from build123d import *

# Parameters (mm, degrees)
SALIENTE_EXTRUIR1_DEPTH = 5
REDONDEO1_R             = 10
CROQUIS2_R              = 1.5
CROQUIS2_W              = 40
CROQUIS2_H              = 20
CORTAR_EXTRUIR1_DEPTH   = 135.669558943
CROQUIS3_W              = 4
CROQUIS3_H              = 14.636342218
CORTAR_EXTRUIR2_DEPTH   = 135.669558943


with BuildPart() as part:
    # Croquis1 → Saliente-Extruir1 (new body)
    with BuildSketch(Plane(origin=(0, 0, 0), x_dir=(1, 0, 0), z_dir=(0, 1, 0))):
        Polygon((-88.1, 42.318171109), (88.1, 42.318171109), (108.1, 22.318171109), (127.75, 22.318171109), (127.75, 7.681828891), (105.75, 7.681828891), (77.75, -42.318171109), (-77.75, -42.318171109), (-105.75, 7.681828891), (-127.75, 7.681828891), (-127.75, 22.318171109), (-108.1, 22.318171109), align=None)
    extrude(amount=SALIENTE_EXTRUIR1_DEPTH)

    # Redondeo1
    redondeo1_edges = [part.edges().sort_by_distance(p)[0] for p in [
        (-88.1, 2.5, -42.318171109),
        (88.1, 2.5, -42.318171109),
        (108.1, 2.5, -22.318171109),
        (105.75, 2.5, -7.681828891),
        (77.75, 2.5, 42.318171109),
        (-77.75, 2.5, 42.318171109),
        (-105.75, 2.5, -7.681828891),
        (-108.1, 2.5, -22.318171109),
    ]]
    fillet(redondeo1_edges, radius=REDONDEO1_R)

    # Croquis2 → Cortar-Extruir1 (cut, through all)
    with BuildSketch(Plane(origin=(0, 5, 0), x_dir=(1, 0, 0), z_dir=(0, 1, 0))):
        with Locations(Location((70, -17.318171109, 0), (0, 0, 270))):
            Circle(CROQUIS2_R)
        with Locations(Location((-70, -17.318171109, 0), (0, 0, 270))):
            Circle(CROQUIS2_R)
        with Locations(Location((-119.996067812, 15, 0), (0, 0, 270))):
            Circle(CROQUIS2_R)
        with Locations(Location((119.996067812, 15, 0), (0, 0, 270))):
            Circle(CROQUIS2_R)
        with Locations(Location((-75, 32.318171109, 0), (0, 0, 270))):
            Circle(CROQUIS2_R)
        with Locations(Location((75, 32.318171109, 0), (0, 0, 270))):
            Circle(CROQUIS2_R)
        with Locations(Location((-10, -22.318171109, 0), (0, 0, 270))):
            Circle(CROQUIS2_R)
        with Locations(Location((10, -22.318171109, 0), (0, 0, 270))):
            Circle(CROQUIS2_R)
        with Locations(Location((-10, -37.318171109, 0), (0, 0, 270))):
            Circle(CROQUIS2_R)
        with Locations(Location((10, -37.318171109, 0), (0, 0, 270))):
            Circle(CROQUIS2_R)
        with Locations(Location((-60, -2.681828891, 0), (0, 0, 270))):
            Circle(CROQUIS2_R)
        with Locations(Location((-10, -2.681828891, 0), (0, 0, 270))):
            Circle(CROQUIS2_R)
        with Locations(Location((-60, 3.318171109, 0), (0, 0, 270))):
            Circle(CROQUIS2_R)
        with Locations(Location((-60, -8.681828891, 0), (0, 0, 270))):
            Circle(CROQUIS2_R)
        with Locations(Location((-10, 3.318171109, 0), (0, 0, 270))):
            Circle(CROQUIS2_R)
        with Locations(Location((-10, -8.681828891, 0), (0, 0, 270))):
            Circle(CROQUIS2_R)
        with Locations((-35, -2.681828891)):
            Rectangle(CROQUIS2_W, CROQUIS2_H)
    extrude(amount=-CORTAR_EXTRUIR1_DEPTH, mode=Mode.SUBTRACT)

    # Croquis3 → Cortar-Extruir2 (cut, through all)
    with BuildSketch(Plane(origin=(0, 5, 0), x_dir=(1, 0, 0), z_dir=(0, 1, 0))):
        with Locations((-125.75, 15)):
            Rectangle(CROQUIS3_W, CROQUIS3_H)
        with Locations((125.75, 15)):
            Rectangle(CROQUIS3_W, CROQUIS3_H)
    extrude(amount=-CORTAR_EXTRUIR2_DEPTH, mode=Mode.SUBTRACT)


solid = part.part
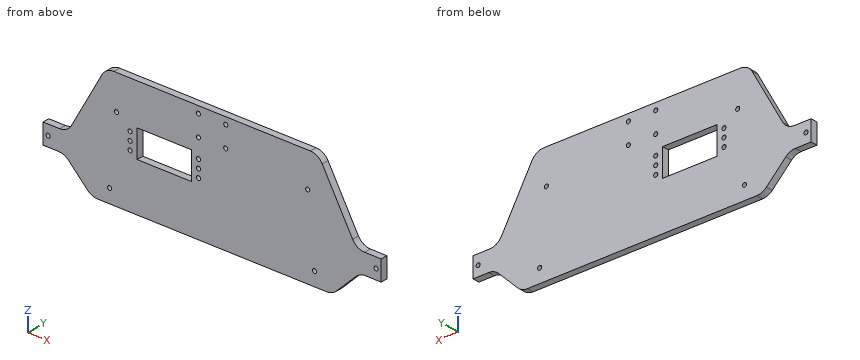
CAD build for the part. Positions are in the model's coordinates, mm. Coordinates: 2 decimals unless noted, no trailing zeros. Write each loop counter-clockwise with the first axis right and the second up, starting at its lowest first coordinate (ties: lowest second). Pieces come first, ordered by that corner, then holes. Notation, with made-up numbers: M 82.5,-10.5 L 98.5,-10.5 A25 cw 98.5,19.5 Z; hole C -15.75,21.5 d11. An arc over 180 degrees is marked long. Answer as a JSON object with one key per item and string values. Group by question number.
1) Saw through at C-C (z = 26). Write the cut outline in (x, y), plus the area to 3 significant figures.
2) Pin check, flat tip, straight feed: pin 1 Ø1.5 at (y, z) = (3.5, 6.5) entering from -X. Stop position of the tip, or through.
3) Saw through at B-B (y = 2.8). Give the number of separate pieces and of enclosed holes in the cut face, plus the area to 3 significant figures.
4) Saw through at D-D (x = -88). Write the cut outline in (y, z).
5) Wall check: line 1 (Z direction, x = -36.5, y = 0.3); line 2 (Z direction, x = 113.5, y = 0.7); line 3 (Z direction, x = 76, y = 3.5). Give the ranges that are in metal, low to high. Write a range as from..to.
6) Saw through at A-A (x = -23). Write the cut outline in (y, z).
Values follow:
{
 "1": {"outline": "M -86.89,0 L 86.89,0 L 86.89,5 L -86.89,5 Z", "area": "869 mm2"},
 "2": {"pin 1": "stops at x = -98.23"},
 "3": {"separate pieces": "1", "enclosed holes": "17", "area": "15,800 mm2"},
 "4": {"outline": "M 0,-41.46 L 5,-41.46 L 5,24.01 L 0,24.01 Z"},
 "5": {"line 1": "z = -42.32..-7.32, 12.68..42.32", "line 2": "z = -22.32..-7.68", "line 3": "z = -42.32..-33.44, -31.2..41.43"},
 "6": {"outline": "M 0,-42.32 L 5,-42.32 L 5,-7.32 L 0,-7.32 Z; M 0,12.68 L 5,12.68 L 5,42.32 L 0,42.32 Z"}
}
